```python
from build123d import *

# Parameters (mm, degrees)
SALIENTE_EXTRUIR1_DEPTH             = 0.5
CROQUIS2_R                          = 0.5
CORTAR_EXTRUIR1_DEPTH               = 0.5
SALIENTE_EXTRUIR2_REACH             = 7.984
SALIENTE_EXTRUIR2_DIRECTION_2_REACH = 7.984


# Read off the part's stored shape, not the designer's step: Diámetro de taladro Ø0.35 (0.35)1
with BuildPart() as part:
    # Croquis1 → Saliente-Extruir1 (new body)
    with BuildSketch(Plane.XY):
        Polygon((-5, 1.75), (-5, -1.75), (-2, -1.75), (-2, -2.75), (2, -2.75), (2, -1.75), (5, -1.75), (5, 1.75), (2, 1.75), (2, 3.25), (-2, 3.25), (-2, 1.75), align=None)
    extrude(amount=SALIENTE_EXTRUIR1_DEPTH)

    # Croquis2 → Cortar-Extruir1 (cut)
    with BuildSketch(Plane.XY.offset(0.5)):
        Circle(CROQUIS2_R)
    extrude(amount=-CORTAR_EXTRUIR1_DEPTH, mode=Mode.SUBTRACT)

    # Saliente-Extruir2: up to this face of the body (flat: up to its plane)
    saliente_extruir2_end = Plane(part.part.faces().sort_by_distance((2, 2.5, 0.25))[0])
    # Croquis3 → Saliente-Extruir2 (add, up to the picked face)
    with BuildSketch(Plane(origin=(0, 0, 0), x_dir=(0, 0, -1), z_dir=(1, 0, 0)), mode=Mode.PRIVATE) as saliente_extruir2_sk1:
        with BuildLine():
            Line((-0.95, 3.25), (-0.95, 3.371997249))
            ThreePointArc((-0.95, 3.371997249), (-0.918397272, 3.493663315), (-0.831578947, 3.584569544))
            ThreePointArc((-0.831578947, 3.584569544), (-0.55232487, 3.707838028), (-0.25, 3.75))
            Line((-0.25, 3.75), (0, 3.75))
            Line((0, 3.75), (0, 3.25))
            Line((0, 3.25), (-0.95, 3.25))
        make_face()
    saliente_extruir2_tool1 = split(extrude(saliente_extruir2_sk1.sketch, amount=SALIENTE_EXTRUIR2_REACH, mode=Mode.PRIVATE), bisect_by=saliente_extruir2_end, keep=Keep.BOTH, mode=Mode.PRIVATE)
    add(saliente_extruir2_tool1.solids().sort_by(Axis((0, 3.476563, 0.431746), (1, 0, 0)))[0])

    # Saliente-Extruir2 direction 2: up to this face of the body (flat: up to its plane)
    saliente_extruir2_direction_2_end = Plane(part.part.faces().sort_by_distance((-2, 2.5, 0.25))[0])
    # Croquis3 → Saliente-Extruir2 direction 2 (add, up to the picked face)
    with BuildSketch(Plane(origin=(0, 0, 0), x_dir=(0, 0, -1), z_dir=(1, 0, 0)), mode=Mode.PRIVATE) as saliente_extruir2_direction_2_sk1:
        with BuildLine():
            Line((-0.95, 3.25), (-0.95, 3.371997249))
            ThreePointArc((-0.95, 3.371997249), (-0.918397272, 3.493663315), (-0.831578947, 3.584569544))
            ThreePointArc((-0.831578947, 3.584569544), (-0.55232487, 3.707838028), (-0.25, 3.75))
            Line((-0.25, 3.75), (0, 3.75))
            Line((0, 3.75), (0, 3.25))
            Line((0, 3.25), (-0.95, 3.25))
        make_face()
    saliente_extruir2_direction_2_tool1 = split(extrude(saliente_extruir2_direction_2_sk1.sketch, amount=-SALIENTE_EXTRUIR2_DIRECTION_2_REACH, mode=Mode.PRIVATE), bisect_by=saliente_extruir2_direction_2_end, keep=Keep.BOTH, mode=Mode.PRIVATE)
    add(saliente_extruir2_direction_2_tool1.solids().sort_by(Axis((0, 3.476563, 0.431746), (-1, 0, 0)))[0])

    # Diámetro de taladro Ø0.35 (0.35)1 outlin → Diámetro de taladro Ø0.35 (0.35)1 (revolve, cut)
    with BuildSketch(Plane(origin=(0, 0.925, 0), x_dir=(0, 1, 0), z_dir=(0, 0, -1))):
        Polygon((0.175, -5), (0.175, -2), (0, -1.894849392), (0, -5), align=None)
        Polygon((0, 5), (0, 1.894849392), (0.175, 2), (0.175, 5), align=None)
    revolve(axis=Axis((0, 0.925, 0), (1, 0, 0)), mode=Mode.SUBTRACT)


solid = part.part
```
Read the model definition and answer for the solid it produces. Units are mm, in the model's axes. A direction names the side the tool comes from. Round coordinates to 2 decimals unless told otherwise and drop trailing zeros. Write each loop counter-clockwise with the first axis right and the second up, starting at its lowest first coordinate (ties: lowest second). Pieces come first, ordered by that corner, then holes. Notation, with made-up numbers: (68, 84.25) -> (114, 84.25) arc R18 cw to (114, 107.25) -> close; hole circle Ø5 at (65.5, -20). An arc over 180 degrees is marked (long way). Answer in a Markdown table with one row per item. Add a question column.
1) Determine the mould class of faces 1 (the face through (-0.108, -0.488, 0.254)), 2 (the face through (0, 1, 0.5)) for opening direction Y: pulls with the +Y half, pulls with the -Y half, needs draft (parallel to the pull), parting line crosses it, or undercut.
2) Which of the six approach directions +Z, -Z, +X, -X, +Y, -Y give full straight-line access (tool end or side, diameter ignored) to faces 3 (the face through (-2, 2.8, 0.3)), 4 (the face through (2, 2.7, 0.3)), 5 (the face through (0, 1, 0))?
3) Given P1, Ø1.8, axis at x = -0.5, y = 0.5, coming from the +Z side, flat-ended and moving along its own axis, determine where the tip first touches the part or whether it passes through.
4) Find section C-C, the plane z = 0.4. Determine the outline of the cut face in (x, y).
5) Consider line 1 (Z direction, x = 1, y = -1.25); line 2 (Y direction, x = 0, z = 0.3). Determine where each line is inside the solid, lowest interval first.
6) Find section D-D, the plane x = -1.5. Determine the outline of the cut face in (y, z) (3 decimals).
7) Find section B-B, the plane x = 0. Determine the outline of the cut face in (y, z) (3 decimals), and give its area (3 significant figures).
8) Find section A-A, the plane y = 0. Determine the outline of the cut face in (x, z).
Findings below:
| question | item | result |
|---|---|---|
| 1 | face 1 | undercut |
| 1 | face 2 | needs draft |
| 2 | face 3 | +Z, -Z, -X, +Y |
| 2 | face 4 | +Z, -Z, +X, +Y |
| 2 | face 5 | -Z, +X, -X, +Y, -Y |
| 3 | P1 | z = 0.5 |
| 4 | outline | (-5, -1.75) -> (-2, -1.75) -> (-2, -2.75) -> (2, -2.75) -> (2, -1.75) -> (5, -1.75) -> (5, 1.75) -> (2, 1.75) -> (2, 3.74) -> (-2, 3.74) -> (-2, 1.75) -> (-5, 1.75) -> close; hole circle Ø1 at (0, 0) |
| 5 | line 1 | 0 to 0.5 |
| 5 | line 2 | -2.75 to -0.5, 0.5 to 3.75 |
| 6 | outline | (-2.75, 0) -> (3.75, 0) -> (3.75, 0.25) arc R1.105 ccw to (3.585, 0.832) arc R0.25 ccw to (3.372, 0.95) -> (3.25, 0.95) -> (3.25, 0.5) -> (-2.75, 0.5) -> close |
| 7 | outline | (-2.75, 0) -> (-0.5, 0) -> (-0.5, 0.5) -> (-2.75, 0.5) -> close; (0.5, 0) -> (3.75, 0) -> (3.75, 0.25) arc R1.105 ccw to (3.585, 0.832) arc R0.25 ccw to (3.372, 0.95) -> (3.25, 0.95) -> (3.25, 0.5) -> (0.5, 0.5) -> close |
| 7 | area | 2.92 mm² |
| 8 | outline | (-5, 0) -> (-0.5, 0) -> (-0.5, 0.5) -> (-5, 0.5) -> close; (0.5, 0) -> (5, 0) -> (5, 0.5) -> (0.5, 0.5) -> close |
